Work out the finished part from the listing and answer in its coordinate system (mm). Round coordinates to 2 decimals unless told otherwise and drop trailing zeros. Order: outer loops, then holes, each group sorted by start corner. A loop starts at its lowest first (then second) coordinate and runs counter-clockwise, first axis right, second up. Notation, with made-up numbers: (-16.75, 38) - (40.25, 38) arc R20 cw to (40.25, 76) - close; hole circle Ø4 at (-31, 23.5). An arc over 180 degrees is marked (long way). Answer in a Markdown table with one row per item.
Autodesk Inventor part; units mm, degrees
ref_plane "YZ Plane" through (0, 0, 0) normal (1, 0, 0) x (0, 1, 0)
ref_plane "XZ Plane" through (0, 0, 0) normal (0, 1, 0) x (-1, 0, 0)
ref_plane "XY Plane" through (0, 0, 0) normal (0, 0, 1) x (1, 0, 0)
sketch "Sketch1" plane through (0, 0, 0) normal (0, 0, 1) x (1, 0, 0)
  circle A0 centre (0.7751, 127) radius 2.0955
  circle A1 centre (0.7751, 139.7) radius 2.0955
  circle A2 centre (0.7751, 152.4) radius 2.0955
  circle A3 centre (51.5751, 152.4) radius 2.0955
  circle A4 centre (51.5751, 139.7) radius 2.0955
  line L0 (57.9251, 139.7) -> (57.9251, 152.4)
  line L1 (-5.5749, 127) -> (-5.5749, 197.5923)
  line L2 (57.9251, 152.4) -> (57.9251, 163.3023)
  line L3 (-0.7663, 200.3149) -> (56.3837, 166.0249)
  spline S0 degree 4 poles (56.3837, 166.0249) (56.7408, 165.8106) (57.455, 165.3821) (57.9251, 164.5517) (57.9251, 163.7188) (57.9251, 163.3023) knots 0 0 0 0 0 0.5 1 1 1 1 1
  spline S1 degree 4 poles (-0.7663, 200.3149) (-1.5089, 200.7604) (-2.9939, 201.6514) (-5.5749, 200.1901) (-5.5749, 198.4583) (-5.5749, 197.5923) knots 0 0 0 0 0 0.5 1 1 1 1 1
  line L4 (7.1251, 147.6375) -> (8.9582, 151.7525) construction
  line L5 (8.9582, 151.7525) -> (16.6389, 151.7525) construction
  line L6 (16.6389, 151.7525) -> (25.4, 151.7525) construction
  line L7 (25.4, 151.7525) -> (33.3375, 150.3172) construction
  line L8 (33.3375, 150.3172) -> (39.6875, 147.6375) construction
  line L9 (39.6875, 147.6375) -> (45.2251, 139.7) construction
  spline S2 degree 4 poles (7.1251, 147.6375) (8.9582, 151.7525) (16.6389, 151.7525) (25.4, 151.7525) (33.3375, 150.3172) (39.6875, 147.6375) (45.2251, 139.7) knots 1 1 1 1 1 2 3 4 4 4 4 4
  arc A5 (-5.5749, 127) -> (7.1251, 127) centre (0.7751, 127) ccw
  line L10 (7.1251, 127) -> (7.1251, 144.4625)
  spline S3 degree 4 poles (7.1251, 144.4625) (7.1251, 144.8594) (7.1251, 145.6531) (6.6738, 146.4787) (6.9567, 147.2593) (7.1251, 147.6375) knots 0 0 0 0 0 0.5 1 1 1 1 1
  arc A6 (47.3211, 134.9856) -> (57.9251, 139.7) centre (51.5751, 139.7) ccw
  spline S4 degree 4 poles (47.3211, 134.9856) (46.8217, 135.4363) (45.9501, 136.4787) (46.3422, 138.0988) (45.5975, 139.1663) (45.2251, 139.7) knots 0 0 0 0 0 0.5 1 1 1 1 1
  circle A7 centre (1.1822, 191.2221) radius 2.0955
  circle A8 centre (27.4016, 175.4904) radius 2.0955
  circle A9 centre (43.5997, 165.7716) radius 2.0955
  circle A10 centre (1.1822, 171.45) radius 2.0955
  point P0 (0, 0)
  point P1 (-5.5749, 203.2)
  point P2 (57.9251, 165.1)
  dimension "d7" = 50.8
  dimension "d8" = 12.7
  dimension "d10" = 6.35
  dimension "d13" = 4.191
  dimension "d14" = 4.191
  dimension "d15" = 4.191
  dimension "d16" = 4.191
  dimension "d17" = 4.191
  dimension "d18" = 4.191
  dimension "d19" = 4.191
  dimension "d20" = 4.191
  dimension "d21" = 4.191
extrude "Extrusion1" add sketch "Sketch1" along normal blind 1.524
properties part number "funnel"
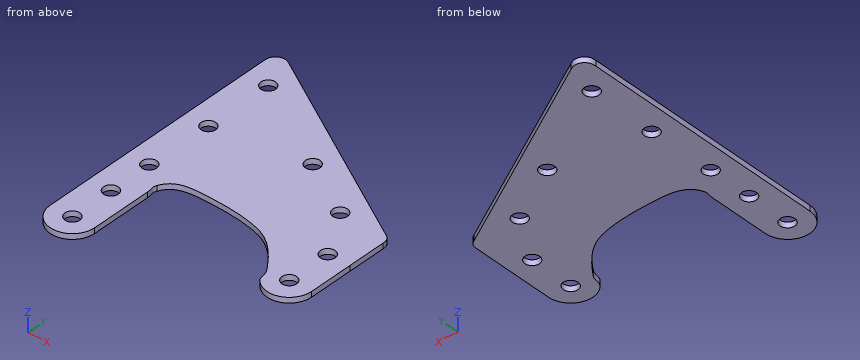
1) Find the intervals of material crossed by probe 1 along X at (y, z) = (152.4, 0.85); probe 2 along Y at (x, z) = (2.5, 1); probe 3 along X at (y, z) = (138, 1), in increasing order. Write a range as from..to.
Filled in:
| item | result |
|---|---|
| probe 1 | x = -5.57..-1.32, 2.87..49.48, 53.67..57.93 |
| probe 2 | y = 120.89..125.81, 128.19..138.51, 140.89..151.21, 153.59..169.82, 173.08..189.59, 192.85..198.36 |
| probe 3 | x = -5.57..-0.45, 2..7.13, 46.04..50.35, 52.8..57.69 |
2) This flat-tipped pin is pushed along its axis until it touches: pin 1 (0.5 mm diameter, centred on y = 138.5, z = 1, fed in from +X). Where does it stop, or does it pass through?
Filled in:
| item | result |
|---|---|
| pin 1 | stops at x = 57.85 |
3) Find section B-B, the plane x = 1.5. Give the vertices of the cut face in (y, z), then the cut area to 3 significant figures.
Filled in:
| item | result |
|---|---|
| outline | (120.69, 0) - (125.03, 0) - (125.03, 1.52) - (120.69, 1.52) - close; (128.97, 0) - (137.73, 0) - (137.73, 1.52) - (128.97, 1.52) - close; (141.67, 0) - (150.43, 0) - (150.43, 1.52) - (141.67, 1.52) - close; (154.37, 0) - (169.38, 0) - (169.38, 1.52) - (154.37, 1.52) - close; (173.52, 0) - (189.15, 0) - (189.15, 1.52) - (173.52, 1.52) - close; (193.29, 0) - (198.96, 0) - (198.96, 1.52) - (193.29, 1.52) - close |
| area | 88.7 mm^2 |
4) Find section A-A, the plane y = 126. Give the vertices of the cut face in (x, z).
Filled in:
| item | result |
|---|---|
| outline | (-5.5, 0) - (-1.07, 0) - (-1.07, 1.52) - (-5.5, 1.52) - close; (2.62, 0) - (7.05, 0) - (7.05, 1.52) - (2.62, 1.52) - close |
5) Find section C-C, the plane z = 0.9. Give the number of separate pieces and of enclosed holes in the cut face, then the cut area to 3 significant figures.
Filled in:
| item | result |
|---|---|
| separate pieces | 1 |
| enclosed holes | 9 |
| area | 2,610 mm^2 |
6) Find section D-D, the plane y = 171.45. Give the vertices of the cut face in (x, z), then the cut area to 3 significant figures.
Filled in:
| item | result |
|---|---|
| outline | (-5.57, 0) - (-0.91, 0) - (-0.91, 1.52) - (-5.57, 1.52) - close; (3.28, 0) - (47.34, 0) - (47.34, 1.52) - (3.28, 1.52) - close |
| area | 74.3 mm^2 |
